```python
from build123d import *

# Parameters (mm, degrees)
SKETCH3_R          = 1.5
CUT_EXTRUDE1_DEPTH = 8.858116823
SKETCH4_R          = 3.5
CUT_EXTRUDE2_DEPTH = 5


with BuildPart() as part:
    # Sketch2 → Revolve1 (revolve)
    with BuildSketch(Plane.XY):
        Polygon((0, 0), (6, 0), (7.5, 7.858116823), (0, 7.858116823), align=None)
    revolve(axis=Axis((0, 0, 0), (0, 1, 0)))

    # Sketch3 → Cut-Extrude1 (cut, through all)
    with BuildSketch(Plane(origin=(0, 0, 0), x_dir=(-1, 0, 0), z_dir=(0, -1, 0))):
        Circle(SKETCH3_R)
    extrude(amount=-CUT_EXTRUDE1_DEPTH, mode=Mode.SUBTRACT)

    # Sketch4 → Cut-Extrude2 (cut)
    with BuildSketch(Plane(origin=(0, 0, 0), x_dir=(-1, 0, 0), z_dir=(0, -1, 0))):
        Circle(SKETCH4_R)
    extrude(amount=-CUT_EXTRUDE2_DEPTH, mode=Mode.SUBTRACT)


solid = part.part
```
Read the model definition and answer for the solid it produces. Units are mm, in the model's axes. A direction names the side the tool comes from. Give positions to 0.01 mm unless a question says otherwise; leave off trailing zeros. Write each loop counter-clockwise with the first axis right and the second up, starting at its lowest first coordinate (ties: lowest second). Pieces come first, ordered by that corner, then holes. Notation, with made-up numbers: (47, -8.75) -> (74, -8.75) arc R15 cw to (74, 20.25) -> close; hole circle Ø3 at (83, 15.5). An arc over 180 degrees is marked (long way). Answer in a Markdown table with one row per item.
1) Straight lines are drawn through the part: line 1 (Y direction, x = 2.5, z = 1.75); line 2 (Z direction, x = -3, y = 4.5); line 3 (X direction, y = 6.5, z = -0.5). For each, find the intervals that lie inside material, in ascending order. Write a range as [from, to].
Results list:
| item | result |
|---|---|
| line 1 | [5, 7.86] |
| line 2 | [-6.17, -1.8], [1.8, 6.17] |
| line 3 | [-7.22, -1.41], [1.41, 7.22] |
2) Section A-A on z = 0 is taken. Give the vertices of the cut face in (x, y).
Results list:
| item | result |
|---|---|
| outline | (-7.5, 7.86) -> (-6, 0) -> (-3.5, 0) -> (-3.5, 5) -> (-1.5, 5) -> (-1.5, 7.86) -> close; (1.5, 5) -> (3.5, 5) -> (3.5, 0) -> (6, 0) -> (7.5, 7.86) -> (1.5, 7.86) -> close |
3) A tool of negligible diameter and unlimited length cuts with its end or side. For faces 1 (the flat face through (0, 5, 2)), 2 (the cylindrical face through (1.5, 6.41, -0.07)), from which of +Z, -Z, +X, -X, +Y, -Y can it reach the whole face along a straight path? Write none if from no direction.
Results list:
| item | result |
|---|---|
| face 1 | -Y |
| face 2 | +Y, -Y |
4) Each of these flat-tipped pins is pushed along its axis until it touches: pin 1 Ø3 at (x, z) = (4, -0.5) entering from -Y; pin 2 Ø5 at (x, z) = (0, 0) entering from -Y. Where does it stop, or does it pass through?
Results list:
| item | result |
|---|---|
| pin 1 | y = 0 |
| pin 2 | y = 5 |
5) Section B-B on x = 0 is taken. Give the vertices of the cut face in (y, z).
Results list:
| item | result |
|---|---|
| outline | (0, -6) -> (7.86, -7.5) -> (7.86, -1.5) -> (5, -1.5) -> (5, -3.5) -> (0, -3.5) -> close; (0, 3.5) -> (5, 3.5) -> (5, 1.5) -> (7.86, 1.5) -> (7.86, 7.5) -> (0, 6) -> close |
6) Section C-C on y = 6.25 is taken. Give the vertices of the cut face in (x, z).
Results list:
| item | result |
|---|---|
| outline | circle Ø14.39 at (0, 0); hole circle Ø3 at (0, 0) |
7) Determine the mould class of faces 3 (the cylindrical face through (-3.233, 2.465, 1.341)), 4 (the flat face through (-3, 0, 3)), 5 (the conical face through (-0.858, 3.111, -6.538)) for opening direction Z: released by +Z, released by -Z, zero draft, split by the parting line, or undercut.
Results list:
| item | result |
|---|---|
| face 3 | undercut |
| face 4 | zero draft |
| face 5 | split by the parting line |
